```python
from build123d import *

# Parameters (mm, degrees)
IZIM1_R                     = 350
Y_KSEKLIK_EKSTR_ZYON2_DEPTH = 5


with BuildPart() as part:
    # Çizim1 → Yükseklik-Ekstrüzyon2 (new body)
    with BuildSketch(Plane(origin=(0, 0, 0), x_dir=(1, 0, 0), z_dir=(0, 1, 0))):
        with Locations(Location((0, 0, 0), (0, 0, 270))):
            Circle(IZIM1_R)
        with BuildLine():
            Line((7.5, -150), (7.5, -99.718353376))
            ThreePointArc((7.5, -99.718353376), (100, 0), (7.5, 99.718353376))
            Line((7.5, 99.718353376), (7.5, 150))
            Line((7.5, 150), (-7.5, 150))
            Line((-7.5, 150), (-7.5, 99.718353376))
            ThreePointArc((-7.5, 99.718353376), (-100, 0), (-7.5, -99.718353376))
            Line((-7.5, -99.718353376), (-7.5, -150))
            Line((-7.5, -150), (7.5, -150))
        make_face(mode=Mode.SUBTRACT)
        with BuildLine():
            Line((239.321958875, 125), (282.655877073, 150.018849336))
            ThreePointArc((282.655877073, 150.018849336), (320, 0), (282.655877073, -150.018849336))
            Line((282.655877073, -150.018849336), (239.321958875, -125))
            ThreePointArc((239.321958875, -125), (270, 0), (239.321958875, 125))
        make_face(mode=Mode.SUBTRACT)
    extrude(amount=Y_KSEKLIK_EKSTR_ZYON2_DEPTH)


solid = part.part
```
Geometry check sheet. Reference: the model listing, model coordinates, mm. A direction names the side the tool comes from. Coordinates: 2 decimals unless noted, no trailing zeros. Order: outer loops, then holes, each group sorted by start corner. A loop starts at its lowest first (then second) coordinate and runs counter-clockwise, first axis right, second up.
Q1. Sectioned sample at C-C on y = 2.15. Record the cut outline in (x, z).
Reply:
outline: circle Ø700 at (0, 0); hole (-7.5, -150) - (7.5, -150) - (7.5, -99.72) arc R100 ccw to (7.5, 99.72) - (7.5, 150) - (-7.5, 150) - (-7.5, 99.72) arc R100 ccw to (-7.5, -99.72) - close; hole (239.32, -125) - (282.66, -150.02) arc R320 ccw to (282.66, 150.02) - (239.32, 125) arc R270 cw to start
Q2. Depth check by flat-ended pin: pin 1 Ø1 at (y, z) = (2, 179.5) entering from -X; pin 2 Ø2.5 at (x, y) = (-1.5, 3) entering from +Z; pin 3 Ø2.5 at (y, z) = (2, -113) entering from +X; pin 4 Ø12 at (x, z) = (0.5, -134.5) entering from +Y. Enter the tip coordinate at first touch or a pass-through.
Reply:
pin 1: stops at x = -300.76
pin 2: stops at z = 350
pin 3: stops at x = 331.68
pin 4: passes through
Q3. Thickness scan on probe 1 along X at (y, z) = (1.1, -116); probe 2 along Z at (x, y) = (242, 1.75); probe 3 along X at (y, z) = (4.2, 132.5). Record the ranges inside material, lowest first.
Reply:
probe 1: x = -330.22 to -7.5, 7.5 to 243.81, 298.23 to 330.22
probe 2: z = -252.86 to -126.55, -119.73 to 119.73, 126.55 to 252.86
probe 3: x = -323.95 to -7.5, 7.5 to 252.31, 291.28 to 323.95
Q4. Sectioned sample at D-D on x = 91. Record the cut outline in (y, z).
Reply:
outline: (0, -337.96) - (5, -337.96) - (5, -41.46) - (0, -41.46) - close; (0, 41.46) - (5, 41.46) - (5, 337.96) - (0, 337.96) - close
Q5. Sectioned sample at A-A on z = 0. Record the cut outline in (x, y).
Reply:
outline: (-350, 0) - (-100, 0) - (-100, 5) - (-350, 5) - close; (100, 0) - (270, 0) - (270, 5) - (100, 5) - close; (320, 0) - (350, 0) - (350, 5) - (320, 5) - close
Q6. Tool access check on faces 4 (the face through (261.292, 2.465, 137.685)), 5 (the face through (-73, 5, 73)). Record the directions out of +Z, -Z, +X, -X, +Y, -Y that give a thin tool (end or side, any length) a straight path to the whole face; none if there is none.
Reply:
face 4: +Y, -Y
face 5: +Z, -Z, +X, -X, +Y
Q7. Draft check along X on faces 1 (the face through (-73, 0, 73)), 2 (the face through (-99.98, 2.46, -2.09)), 3 (the face through (347.022, 2.465, -45.563)). Enter one of: released by +X, released by -X, zero draft, split by the parting line, or undercut.
Reply:
face 1: zero draft
face 2: undercut
face 3: split by the parting line
Q8. Sectioned sample at B-B on x = -40. Record the cut outline in (y, z), and give its area (3 significant figures).
Reply:
outline: (0, -347.71) - (5, -347.71) - (5, -91.65) - (0, -91.65) - close; (0, 91.65) - (5, 91.65) - (5, 347.71) - (0, 347.71) - close
area: 2,560 mm2
